Design review of the part built by this model. Coordinates are the model's own, in mm. A direction names the side the tool comes from. Round coordinates to 2 decimals unless told otherwise and drop trailing zeros. Loops run counter-clockwise (first coordinate to the right, second up) from the corner with the lowest first, then second, coordinate; pieces in that order, holes last. Notation, with made-up numbers: (-19, -15.75) -> (33, -15.75) arc R6 cw to (33, -8.75) -> close; hole circle Ø4 at (80, 24.5). An arc over 180 degrees is marked (long way). Use a Markdown table: item, result. Add a question column.
from build123d import *
from build123d.topology import SkipClean

# Parameters (mm, degrees)
SKETCH1_R               = 32.5
SKETCH1_W               = 120.65
SKETCH1_H               = 50.8
BOSS_EXTRUDE2_DEPTH     = 6.35
BOSS_EXTRUDE3_START     = 6.35
SKETCH1_3_R             = 32.5
BOSS_EXTRUDE3_DEPTH     = 25.4
SKETCH2_R               = 3.175
CUT_EXTRUDE1_DEPTH      = 180.118124432
CUT_EXTRUDE1_DEPTH_BACK = 180.118124432
SKETCH3_R               = 6.35
CUT_EXTRUDE2_DEPTH      = 25.4
FILLET1_R               = 12.7
SKETCH5_R               = 3.175
SKETCH5_R_2             = 32.5
BOSS_EXTRUDE6_DEPTH     = 19.05
SKETCH6_R               = 32.5
SKETCH6_R_2             = 27.5
BOSS_EXTRUDE7_DEPTH     = 2.54


with BuildPart() as part:
    # Sketch1 → Boss-Extrude2 (new body)
    with BuildSketch(Plane.XY):
        with BuildLine():
            Line((32.171066193, 31.75), (171.45, 31.75))
            Line((171.45, 31.75), (171.45, 25.4))
            Line((171.45, 25.4), (50.8, 25.4))
            Line((50.8, 25.4), (50.8, -25.4))
            Line((50.8, -25.4), (171.45, -25.4))
            Line((171.45, -25.4), (171.45, -31.75))
            Line((171.45, -31.75), (32.171066193, -31.75))
            ThreePointArc((32.171066193, -31.75), (-45.2, 0), (32.171066193, 31.75))
        make_face()
        Circle(SKETCH1_R, mode=Mode.SUBTRACT)
        with Locations((111.125, 0)):
            Rectangle(SKETCH1_W, SKETCH1_H)
    extrude(amount=BOSS_EXTRUDE2_DEPTH)

    # Sketch1<3> → Boss-Extrude3 (add)
    with BuildSketch(Plane.XY.offset(BOSS_EXTRUDE3_START)):
        with BuildLine():
            Line((32.171066193, 31.75), (171.45, 31.75))
            Line((171.45, 31.75), (171.45, 25.4))
            Line((171.45, 25.4), (50.8, 25.4))
            Line((50.8, 25.4), (50.8, -25.4))
            Line((50.8, -25.4), (171.45, -25.4))
            Line((171.45, -25.4), (171.45, -31.75))
            Line((171.45, -31.75), (32.171066193, -31.75))
            ThreePointArc((32.171066193, -31.75), (-45.2, 0), (32.171066193, 31.75))
        make_face()
        Circle(SKETCH1_3_R, mode=Mode.SUBTRACT)
    extrude(amount=BOSS_EXTRUDE3_DEPTH)

    # Sketch2 → Cut-Extrude1 (cut, two sides)
    with BuildSketch(Plane.XY.offset(6.35)) as cut_extrude1_sk:
        with Locations((60.325, 15.875)):
            Circle(SKETCH2_R)
        with Locations((161.925, 15.875)):
            Circle(SKETCH2_R)
        with Locations((161.925, -15.875)):
            Circle(SKETCH2_R)
        with Locations((60.325, -15.875)):
            Circle(SKETCH2_R)
        with Locations((27.471098449, 27.471098449)):
            Circle(SKETCH2_R)
        with Locations((27.471098449, -27.471098449)):
            Circle(SKETCH2_R)
        with Locations((-27.471098449, -27.471098449)):
            Circle(SKETCH2_R)
        with Locations((-27.471098449, 27.471098449)):
            Circle(SKETCH2_R)
    extrude(amount=CUT_EXTRUDE1_DEPTH, mode=Mode.SUBTRACT)
    extrude(cut_extrude1_sk.sketch, amount=-CUT_EXTRUDE1_DEPTH_BACK, mode=Mode.SUBTRACT)

    # Sketch3 → Cut-Extrude2 (cut)
    with BuildSketch(Plane.XY.offset(31.75)):
        with Locations((55.290128061, 20.909871939)):
            Circle(SKETCH3_R)
        with Locations((55.290128061, -20.909871939)):
            Circle(SKETCH3_R)
    extrude(amount=-CUT_EXTRUDE2_DEPTH, mode=Mode.SUBTRACT)

    # Fillet1
    fillet1_edges = [part.edges().sort_by_distance(p)[0] for p in [
        (32.171066193, -31.75, 15.875),
        (32.171066193, 31.75, 15.875),
    ]]
    fillet(fillet1_edges, radius=FILLET1_R)

    # Sketch5 → Boss-Extrude6 (add)
    with SkipClean():  # the faces are left unmerged after this step: merging them gives an invalid solid
        with BuildSketch(Plane(origin=(0, 0, 0), x_dir=(-1, 0, 0), z_dir=(0, 0, -1))):
            with BuildLine():
                ThreePointArc((-28.964426695, -34.700172712), (45.2, 0), (-28.964426695, 34.700172712))
                ThreePointArc((-28.964426695, 34.700172712), (-45.2, 0), (-28.964426695, -34.700172712))
            make_face()
            with Locations(Location((-27.471098449, -27.471098449, 0), (0, 0, 180))):
                Circle(SKETCH5_R, mode=Mode.SUBTRACT)
            with Locations(Location((27.471098449, -27.471098449, 0), (0, 0, 180))):
                Circle(SKETCH5_R, mode=Mode.SUBTRACT)
            with Locations(Location((27.471098449, 27.471098449, 0), (0, 0, 180))):
                Circle(SKETCH5_R, mode=Mode.SUBTRACT)
            with Locations(Location((-27.471098449, 27.471098449, 0), (0, 0, 180))):
                Circle(SKETCH5_R, mode=Mode.SUBTRACT)
            Circle(SKETCH5_R_2, mode=Mode.SUBTRACT)
        extrude(amount=BOSS_EXTRUDE6_DEPTH)

    # Sketch6 → Boss-Extrude7 (add)
    with SkipClean():  # the faces are left unmerged after this step: merging them gives an invalid solid
        with BuildSketch(Plane(origin=(0, 0, -19.05), x_dir=(-1, 0, 0), z_dir=(0, 0, -1))):
            Circle(SKETCH6_R)
            Circle(SKETCH6_R_2, mode=Mode.SUBTRACT)
        extrude(amount=-BOSS_EXTRUDE7_DEPTH)


solid = part.part
1. Consider section C-C on z = 24. State the section outline as (x, y) points (3 decimals).
2. To check wall thickness, follow probe 1 along Y at (x, z) = (99, 29.5); probe 2 along Y at (x, z) = (-30, 23.5); probe 3 along Y at (x, z) = (0, -8). State the ranges of each line that lie inside material, in increasing order. Write a range as from..to.
3. For faces 1 (the face through (50.8, 0, 19)), 2 (the face through (27, 7, -16.51)), 3 (the face through (103, 31.75, 16)), list the 3-axis set-ups (+Z, -Z, +X, -X, +Y, -Y) from which the entire face can be reached by the end or side of a thin tool; tool diameter is ignored.
4. Mouldability with a two-part tool opening along Y and no side actions: class faces 4 (the face through (40, 0, 31.75)), 5 (the face through (50.7, -25.3, 19.2)), 6 (the face through (105, -31.75, 16)) as +Y half, -Y half, draft (parallel to the pull), parting line (faces both ways), or undercut.
5. Consider section A-A on x = 0. State the section outline as (y, z) points.
6. Consider section B-B on y = 0. State the section outline as (x, z) points, plus the area to 3 significant figures.
7. Consider section D-D on x = 142.5. State the section outline as (y, z) points, plus the area to 3 significant figures.
8. Insertion check: P1, Ø15, axis at x = 91.5, y = -1, coming from the +Z side; P2, Ø0.9, axis at x = 50.5, y = -21, coming from the +Z side; P3, Ø2, axis at x = 69.5, z = 21, coming from the -Y side; P4, Ø5.5, axis at x = -27.47, y = 27.47, coming from the -Z side. Each pin has a flat end and moves straight along its axis. Give the tip position at first contact, or say it passes through.
Verdict:
| question | item | result |
|---|---|---|
| 1 | outline | (28.964, -34.7) arc R12.7 cw to (37.103, -31.75) -> (171.45, -31.75) -> (171.45, -25.4) -> (59.78, -25.4) arc R6.35 cw to (50.8, -16.42) -> (50.8, 16.42) arc R6.35 cw to (59.78, 25.4) -> (171.45, 25.4) -> (171.45, 31.75) -> (37.103, 31.75) arc R12.7 cw to (28.964, 34.7) arc R45.2 ccw (long way) to start; hole circle Ø65 at (0, 0); hole circle Ø6.35 at (-27.471, -27.471); hole circle Ø6.35 at (-27.471, 27.471); hole circle Ø6.35 at (27.471, -27.471); hole circle Ø6.35 at (27.471, 27.471) |
| 2 | probe 1 | y = -31.75..-25.4, 25.4..31.75 |
| 2 | probe 2 | y = -33.81..-29.39, -25.55..-12.5, 12.5..25.55, 29.39..33.81 |
| 2 | probe 3 | y = -45.2..-32.5, 32.5..45.2 |
| 3 | face 1 | +Z, +X |
| 3 | face 2 | +Z |
| 3 | face 3 | +Z, -Z, +X, +Y |
| 4 | face 4 | draft |
| 4 | face 5 | undercut |
| 4 | face 6 | -Y half |
| 5 | outline | (-45.2, -19.05) -> (-27.5, -19.05) -> (-27.5, -16.51) -> (-32.5, -16.51) -> (-32.5, 31.75) -> (-45.2, 31.75) -> close; (27.5, -19.05) -> (45.2, -19.05) -> (45.2, 31.75) -> (32.5, 31.75) -> (32.5, -16.51) -> (27.5, -16.51) -> close |
| 6 | outline | (-45.2, -19.05) -> (-27.5, -19.05) -> (-27.5, -16.51) -> (-32.5, -16.51) -> (-32.5, 31.75) -> (-45.2, 31.75) -> close; (27.5, -19.05) -> (45.2, -19.05) -> (45.2, 0) -> (171.45, 0) -> (171.45, 6.35) -> (50.8, 6.35) -> (50.8, 31.75) -> (32.5, 31.75) -> (32.5, -16.51) -> (27.5, -16.51) -> close |
| 6 | area | 2,260 mm² |
| 7 | outline | (-31.75, 0) -> (31.75, 0) -> (31.75, 31.75) -> (25.4, 31.75) -> (25.4, 6.35) -> (-25.4, 6.35) -> (-25.4, 31.75) -> (-31.75, 31.75) -> close |
| 7 | area | 726 mm² |
| 8 | P1 | stops at z = 6.35 |
| 8 | P2 | stops at z = 6.35 |
| 8 | P3 | stops at y = -31.75 |
| 8 | P4 | passes through |
